Input: part model. Units: mm. Frame: model coordinates. Coordinates: 2 decimals unless noted, no trailing zeros. Loops run counter-clockwise (first coordinate to the right, second up) from the corner with the lowest first, then second, coordinate; pieces in that order, holes last.
Item 1: Contact query for a flat-ended pin moving along its axis: P1, Ø0.6, axis at x = 3.5, y = 5, coming from the +Z side. Output: stop coordinate, or through.
Item 2: Pull-direction query (X, two-part tool) for faces 1 (the flat face through (14.5, 22, 3)), 2 (the flat face through (-0.5, 22, 3)), 3 (the conical face through (2.16, 10.98, 2.83)), 4 (the flat face through (7, 23, 0)); classes: released by +X, released by -X, zero draft, split by the parting line, or undercut.
Item 3: Section C-C on z = 1.75. Give the number of separate pieces and of enclosed holes in the cut face, and give its area (3 significant figures).
Item 4: Ray query, line 1 along X through (y, z) = (5, 2.75); line 2 along X through (y, z) = (18.5, 5.5). Return the intervals inside material, ascending.
Item 5: Section B-B on y = 33. Return loops of the section in (x, z), and give its area (3 significant figures).
```python
from build123d import *

# Parameters (mm, degrees)
ARRAY_X_COUNT = 2
ARRAY_X_PITCH = 7
ARRAY_Y_COUNT = 6
ARRAY_Y_PITCH = 7
BOX_W         = 15
BOX_H         = 45
BOX_DEPTH     = 7
FILLET_R      = 0.5


with BuildPart() as array:
    # Cone → Cone (revolve)
    with BuildSketch(Plane(origin=(3.5, 5, 0), x_dir=(1, 0, 0), z_dir=(0, -1, 0))):
        Polygon((0, 0), (1, 0), (2.75, 6.99), (0, 6.99), align=None)
    revolve(axis=Axis((3.5, 5, 0), (0, 0, 1)))

    # Array X: Array ×2


with BuildPart() as array_1:
    add(array.part)
    with Locations(*[(i * ARRAY_X_PITCH, 0, 0) for i in range(1, ARRAY_X_COUNT)]):
        add(array.part)

    # Array Y: Array ×6


with BuildPart() as array_2:
    add(array_1.part)
    with Locations(*[(0, i * ARRAY_Y_PITCH, 0) for i in range(1, ARRAY_Y_COUNT)]):
        add(array_1.part)


with BuildPart() as array_3:
    # Array placement: moved
    add(array_2.part.moved(Location((0, 0, 0.1))))


with BuildPart() as cut:
    # Box → Box (new body)
    with BuildSketch(Plane(origin=(-0.5, 0, 0), x_dir=(1, 0, 0), z_dir=(0, 0, 1))):
        with Locations((7.5, 22.5)):
            Rectangle(BOX_W, BOX_H)
    extrude(amount=BOX_DEPTH)

    # Fillet
    fillet_edges = [cut.edges().sort_by_distance(p)[0] for p in [
        (-0.5, 0, 3.5),
        (-0.5, 22.5, 7),
        (-0.5, 45, 3.5),
        (-0.5, 22.5, 0),
        (14.5, 0, 3.5),
        (14.5, 22.5, 7),
        (14.5, 45, 3.5),
        (14.5, 22.5, 0),
        (7, 0, 0),
        (7, 0, 7),
        (7, 45, 0),
        (7, 45, 7),
    ]]
    fillet(fillet_edges, radius=FILLET_R)

    # Cut: cut Array
    add(array_3.part, mode=Mode.SUBTRACT)


solid = cut.part
```
Results found:
1. P1: stops at z = 0.1
2. face 1: released by +X
2. face 2: released by -X
2. face 3: undercut
2. face 4: zero draft
3. separate pieces: 1
3. enclosed holes: 12
3. area: 600 mm2
4. line 1: x = -0.5 to 1.84, 5.16 to 8.84, 12.16 to 14.5
4. line 2: x = -0.5 to 1.2, 5.8 to 8.2, 12.8 to 14.5
5. outline: (-0.5, 0.5) arc R0.5 ccw to (0, 0) - (14, 0) arc R0.5 ccw to (14.5, 0.5) - (14.5, 6.5) arc R0.5 ccw to (14, 7) - (13.23, 7) - (11.5, 0.1) - (9.5, 0.1) - (7.77, 7) - (6.23, 7) - (4.5, 0.1) - (2.5, 0.1) - (0.77, 7) - (0, 7) arc R0.5 ccw to (-0.5, 6.5) - close
5. area: 53.3 mm2
